Here's the drawing with two shaded views (mm, measured from the low corner). I have some questions. A direction names the side the tool comes from. Round coordinates to 2 decimals unless told otherwise and drop trailing zeros. Write each loop counter-clockwise with the first axis right and the second up, starting at its lowest first coordinate (ties: lowest second). Pieces come first, ordered by that corner, then holes. Notation, with made-up numbers: M 57.5,36.5 L 66.5,36.5 A23 cw 66.5,51.5 Z; hole C 46.5,-36 d4. An arc over 180 degrees is marked long. Write item = value, one per line. Start each with the question number.
(1) I want a section at D-D (z = 6). List the corners of the cut face in (x, y) for me, and give its area (3 significant figures).
(2) On a 3-axis mill with a long thin cutter (end or side, diameter ignored), from which of +Z, -Z, +X, -X, +Y, -Y can I reach the whole of each face in a straight line? I mean the marked faces 1 and 2. Say none if no direction works.
(3) I want a section at A-A (x = 34). List the corners of the cut face in (y, z) for me, and give its area (3 significant figures).
(4) I want a section at C-C (x = 5.4). List the corners of the cut face in (y, z) for me, and give its area (3 significant figures).
(5) Will these pins go through, and if not, where does the flat tip stop? pin 1 Ø4 at (y, z) = (14.5, 2) entering from +X; pin 2 Ø3.5 at (x, z) = (30, 5) entering from -Y.
(6) I need wall thicknesses on line 1 along X through (y, z) = (10, 3); line 2 along Y through (x, z) = (15, 4.5); line 3 along Y through (x, z) = (35, 3.25). Which ranges of each line are inside material? Lowest first, please.
(7) I want a section at B-B (y = 61). List the corners of the cut face in (x, z) for me, and give its area (3 significant figures).
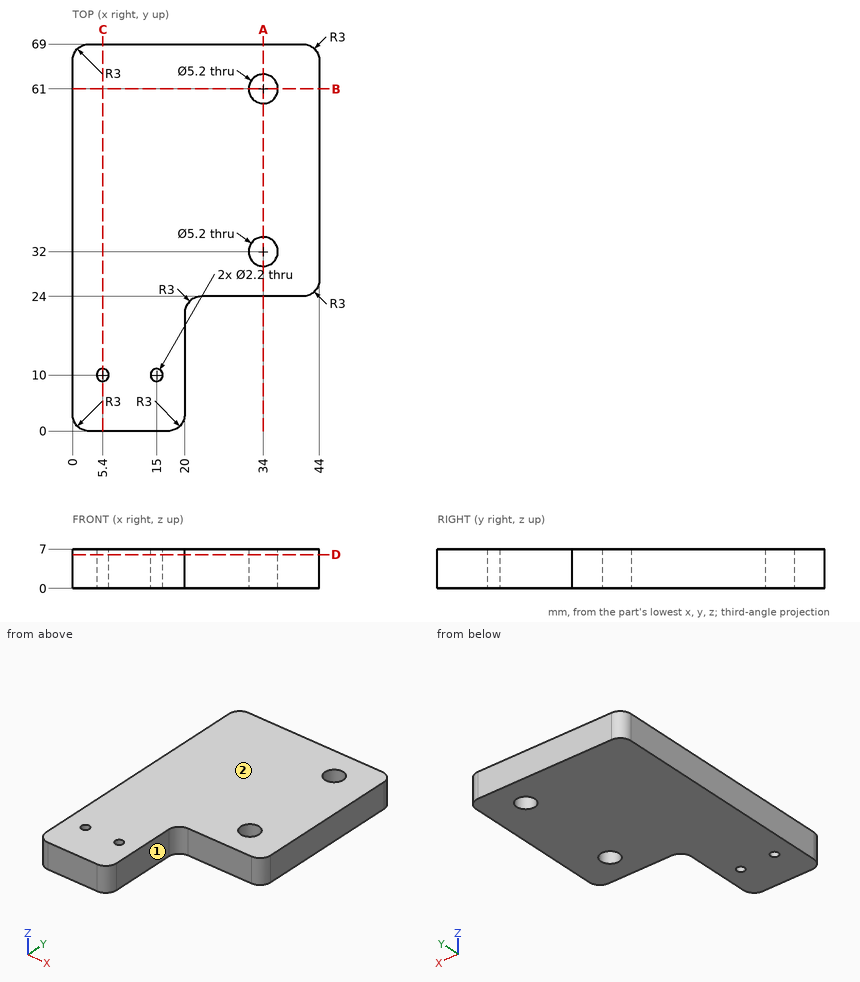
Returned:
q1.outline = M 0,3 A3 ccw 3,0 L 17,0 A3 ccw 20,3 L 20,21 A3 cw 23,24 L 41,24 A3 ccw 44,27 L 44,66 A3 ccw 41,69 L 3,69 A3 ccw 0,66 Z; hole C 5.4,10 d2.2; hole C 15,10 d2.2; hole C 34,32 d5.2; hole C 34,61 d5.2
q1.area = 2,400 mm²
q2.face_1 = +Z, -Z, +X, -Y
q2.face_2 = +Z, +X, -X, +Y, -Y
q3.outline = M 24,0 L 29.4,0 L 29.4,7 L 24,7 Z; M 34.6,0 L 58.4,0 L 58.4,7 L 34.6,7 Z; M 63.6,0 L 69,0 L 69,7 L 63.6,7 Z
q3.area = 242 mm²
q4.outline = M 0,0 L 8.9,0 L 8.9,7 L 0,7 Z; M 11.1,0 L 69,0 L 69,7 L 11.1,7 Z
q4.area = 468 mm²
q5.pin_1 = 20
q5.pin_2 = 24
q6.line_1 = 0 to 4.3, 6.5 to 13.9, 16.1 to 20
q6.line_2 = 0 to 8.9, 11.1 to 69
q6.line_3 = 24 to 29.6, 34.4 to 58.6, 63.4 to 69
q7.outline = M 0,0 L 31.4,0 L 31.4,7 L 0,7 Z; M 36.6,0 L 44,0 L 44,7 L 36.6,7 Z
q7.area = 272 mm²
